```python
from build123d import *

# Parameters (mm, degrees)
F2_DEPTH = 9.5


with BuildPart() as f2:
    # F1 (on Front) → F2 (new body)
    with BuildSketch(Plane.XZ):
        with BuildLine():
            Line((-14.4312179421, -6.5), (30.5, -6.5))
            Line((30.5, -6.5), (30.5, -3.5))
            Line((30.5, -3.5), (2.9580398915, -0.5))
            ThreePointArc((2.9580398915, -0.5), (0, -3), (-2.9580398915, -0.5))
            Line((-2.9580398915, -0.5), (-17.160677935, -0.5))
            Line((-17.160677935, -0.5), (-17.1837798887, -0.5))
            Line((-17.1837798887, -0.5), (-22, -0.5))
            ThreePointArc((-22, -0.5), (-34.6901536634, -12.7), (-47.3803073267, -0.5))
            Line((-47.3803073267, -0.5), (-53.3834679762, -0.5))
            ThreePointArc((-53.3834679762, -0.5), (-37.745644054, -18.4486850066), (-17.1561866279, -6.5))
            Line((-17.1561866279, -6.5), (-16.0312179421, -6.5))
            Line((-16.0312179421, -6.5), (-16.0312179421, -4.9))
            Line((-16.0312179421, -4.9), (-14.4312179421, -4.9))
            Line((-14.4312179421, -4.9), (-14.4312179421, -6.5))
        make_face()
    extrude(amount=F2_DEPTH)


solid = f2.part
```
Source: CAD feature listing. Evaluate the final solid. Frame: model axes, mm. A direction names the side the tool comes from. Round coordinates to 2 decimals unless told otherwise and drop trailing zeros. Order: outer loops, then holes, each group sorted by start corner. A loop starts at its lowest first (then second) coordinate and runs counter-clockwise, first axis right, second up. Notation, with made-up numbers: (-15.75, 23.25) -> (35.25, 23.25) arc R32 ccw to (35.25, 51.25) -> close; hole circle Ø8 at (-29, 54.25). An arc over 180 degrees is marked (long way). One line per item, written item: value. Start each with the question number.
Q1. Access query for faces 4 (the flat face through (-16.031, -5, -6)), 5 (the flat face through (-21, -9.5, -7)), 6 (the flat face through (8, -5, -6.5)). Directions: +Z, -Z, +X, -X, +Y, -Y. A direction counts if a zero-diameter tool reaches every point of the face in a straight line with its end or side. Return the directions, or none.
Q2. Material intervals for probe 1 along Z at (x, y) = (-9.5, -1); probe 2 along X at (y, z) = (-7, -10.5); probe 3 along X at (y, z) = (-7.5, -3.75), sorted ascending.
Q3. Pin query (flat end, axial travel): pin 1 (3 mm diameter, centred on x = 18, y = -4.5, fed in from -Z); pin 2 (1 mm diameter, centred on x = -26, y = -3.5, fed in from -Z); pin 3 (1.8 mm diameter, centred on y = -6, z = -5.5, fed in from -X); pin 4 (2 mm diameter, centred on y = -7, z = -3, fed in from +X). Return the tip coordinate at first contact, or that it passes through.
Q4. Section query B-B (z = -2). Return the cut outline in (x, y).
Q5. Section query A-A (z = -8.5). Return the cut outline in (x, y).
Q6. Section query D-D (x = 7). Return the cut outline in (y, z).
Q7. Draft query along X for faces 1 (the flat face through (30.5, -5, -5)), 2 (the flat face through (-50, -5, -0.5)), 3 (the flat face through (-15, -5, -4.9)). Return one class per face: pulls with the +X half, pulls with the -X half, needs draft (parallel to the pull), parting line crosses it, or undercut.
Q8. Section query C-C (y = -8.5). Return the cut outline in (x, z).
Findings below:
1. face 4: -Z, +Y, -Y
1. face 5: +Z, -Z, +X, -X, -Y
1. face 6: -Z, +X, +Y, -Y
2. probe 1: -6.5 to -0.5
2. probe 2: -50.16 to -41.83, -27.55 to -19.22
2. probe 3: -53.01 to -46.82, -22.56 to 30.5
3. pin 1: z = -6.5
3. pin 2: z = -16.81
3. pin 3: x = -52.82
3. pin 4: x = 30.5
4. outline: (-53.28, -9.5) -> (-47.23, -9.5) -> (-47.23, 0) -> (-53.28, 0) -> close; (-22.15, -9.5) -> (-2.24, -9.5) -> (-2.24, 0) -> (-22.15, 0) -> close; (2.24, -9.5) -> (16.73, -9.5) -> (16.73, 0) -> (2.24, 0) -> close
5. outline: (-51.35, -9.5) -> (-44.13, -9.5) -> (-44.13, 0) -> (-51.35, 0) -> close; (-25.25, -9.5) -> (-18.03, -9.5) -> (-18.03, 0) -> (-25.25, 0) -> close
6. outline: (-9.5, -6.5) -> (0, -6.5) -> (0, -0.94) -> (-9.5, -0.94) -> close
7. face 1: pulls with the +X half
7. face 2: needs draft
7. face 3: undercut
8. outline: (-53.38, -0.5) arc R18.7 ccw to (-17.16, -6.5) -> (-16.03, -6.5) -> (-16.03, -4.9) -> (-14.43, -4.9) -> (-14.43, -6.5) -> (30.5, -6.5) -> (30.5, -3.5) -> (2.96, -0.5) arc R3 cw to (-2.96, -0.5) -> (-22, -0.5) arc R12.7 cw to (-47.38, -0.5) -> close
